Model file for the job. Use its own axes, mm. Face numbers are marked on the shaded views. A direction names the side the tool comes from. Round coordinates to 2 decimals unless told otherwise and drop trailing zeros. Write each loop counter-clockwise with the first axis right and the second up, starting at its lowest first coordinate (ties: lowest second). Pieces come first, ordered by that corner, then holes. Notation, with made-up numbers: (74, 61) - (105, 61) arc R21 ccw to (105, 83) - close; hole circle Ø4 at (68.25, 62). An arc over 180 degrees is marked (long way). One line per item, written item: value.
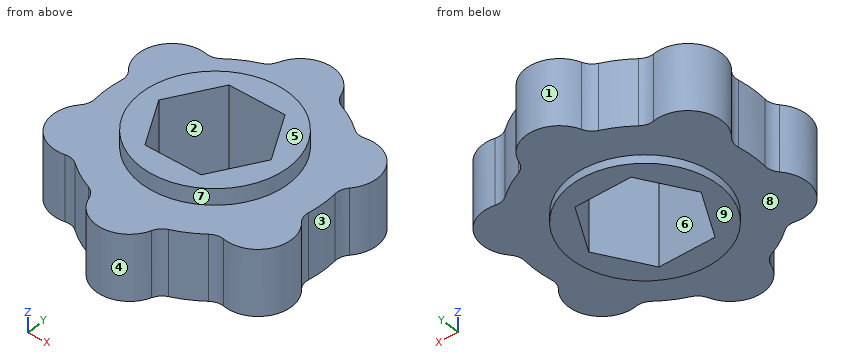
from build123d import *

# Parameters (mm, degrees)
BOSS_EXTRUDE2_DEPTH = 8.509
FILLET1_R           = 2.032
CUT_EXTRUDE1_DEPTH  = 25.900744443
SKETCH7_R           = 9.525
BOSS_EXTRUDE3_DEPTH = 1.0795
BOSS_EXTRUDE4_START = 2.0955
SKETCH8_R           = 9.525
BOSS_EXTRUDE4_DEPTH = 2.0955


with BuildPart() as part:
    # Sketch5 → Boss-Extrude2 (new body)
    with BuildSketch(Plane.XY):
        with BuildLine():
            ThreePointArc((13.895294195, 3.040226179), (15.067976, 8.6995), (9.580560202, 10.513564677))
            ThreePointArc((9.580560202, 10.513564677), (7.112, 12.318345343), (4.314733993, 13.553790856))
            ThreePointArc((4.314733993, 13.553790856), (0, 17.399), (-4.314733993, 13.553790856))
            ThreePointArc((-4.314733993, 13.553790856), (-7.112, 12.318345343), (-9.580560202, 10.513564677))
            ThreePointArc((-9.580560202, 10.513564677), (-15.067976, 8.6995), (-13.895294195, 3.040226179))
            ThreePointArc((-13.895294195, 3.040226179), (-14.224, 0), (-13.895294195, -3.040226179))
            ThreePointArc((-13.895294195, -3.040226179), (-15.067976, -8.6995), (-9.580560202, -10.513564677))
            ThreePointArc((-9.580560202, -10.513564677), (-7.112, -12.318345343), (-4.314733993, -13.553790856))
            ThreePointArc((-4.314733993, -13.553790856), (0, -17.399), (4.314733993, -13.553790856))
            ThreePointArc((4.314733993, -13.553790856), (7.112, -12.318345343), (9.580560202, -10.513564677))
            ThreePointArc((9.580560202, -10.513564677), (15.067976, -8.6995), (13.895294195, -3.040226179))
            ThreePointArc((13.895294195, -3.040226179), (14.224, 0), (13.895294195, 3.040226179))
        make_face()
    extrude(amount=BOSS_EXTRUDE2_DEPTH)

    # Fillet1
    fillet1_edges = [part.edges().sort_by_distance(p)[0] for p in [
        (-4.314733993, 13.553790856, 4.2545),
        (4.314733993, 13.553790856, 4.2545),
        (9.580560202, 10.513564677, 4.2545),
        (13.895294195, 3.040226179, 4.2545),
        (13.895294195, -3.040226179, 4.2545),
        (9.580560202, -10.513564677, 4.2545),
        (4.314733993, -13.553790856, 4.2545),
        (-4.314733993, -13.553790856, 4.2545),
        (-9.580560202, -10.513564677, 4.2545),
        (-13.895294195, -3.040226179, 4.2545),
        (-9.580560202, 10.513564677, 4.2545),
        (-13.895294195, 3.040226179, 4.2545),
    ]]
    fillet(fillet1_edges, radius=FILLET1_R)

    # Sketch6 → Cut-Extrude1 (cut, through all)
    with BuildSketch(Plane.XY.offset(8.509)):
        Polygon((7.405671903, 0), (3.702835951, 6.4135), (-3.702835951, 6.4135), (-7.405671903, 0), (-3.702835951, -6.4135), (3.702835951, -6.4135), align=None)
    extrude(amount=-CUT_EXTRUDE1_DEPTH, mode=Mode.SUBTRACT)

    # Sketch7 → Boss-Extrude3 (add)
    with BuildSketch(Plane(origin=(0, 0, 0), x_dir=(-1, 0, 0), z_dir=(0, 0, -1))):
        with Locations(Location((0, 0, 0), (0, 0, 180))):
            Circle(SKETCH7_R)
        Polygon((-7.405671903, 0), (-3.702835951, 6.4135), (3.702835951, 6.4135), (7.405671903, 0), (3.702835951, -6.4135), (-3.702835951, -6.4135), align=None, mode=Mode.SUBTRACT)
    extrude(amount=BOSS_EXTRUDE3_DEPTH)

    # Sketch8 → Boss-Extrude4 (add)
    with BuildSketch(Plane.XY.offset(8.509).offset(BOSS_EXTRUDE4_START)):
        Circle(SKETCH8_R)
        Polygon((3.702835951, -6.4135), (7.405671903, 0), (3.702835951, 6.4135), (-3.702835951, 6.4135), (-7.405671903, 0), (-3.702835951, -6.4135), align=None, mode=Mode.SUBTRACT)
    extrude(amount=-BOSS_EXTRUDE4_DEPTH)


solid = part.part
1. Tool access for the marked faces 5, 6, 7, 8 and 9: list every direction of +Z, -Z, +X, -X, +Y, -Y with a clear straight run to the whole face (end or side of a thin tool).
Report:
face 5: +Z, +X, -X, +Y, -Y
face 6: +Z, -Z
face 7: +Z
face 8: -Z
face 9: -Z, +X, -X, +Y, -Y
2. Mould opens along Y. For the marked faces 1, 2, 3 and 4 say: released by +Y, released by -Y, zero draft, split by the parting line, or undercut.
Report:
face 1: released by +Y
face 2: undercut
face 3: undercut
face 4: released by -Y
3. Wall check: probe 1 along Z at (x, y) = (6.5, -10); probe 2 along X at (y, z) = (-3, 9.5); probe 3 along X at (y, z) = (-0.5, 0.25). Give the ranges that are in metal, low to high. Write a range as [from, to].
Report:
probe 1: [0, 8.51]
probe 2: [-9.04, -5.67], [5.67, 9.04]
probe 3: [-14.22, -7.12], [7.12, 14.22]
4. Band-saw the part on B-B on x = 0. Write the cut outline in (y, z) (1 decimal).
Report:
outline: (-17.4, 0) - (-9.5, 0) - (-9.5, -1.1) - (-6.4, -1.1) - (-6.4, 10.6) - (-9.5, 10.6) - (-9.5, 8.5) - (-17.4, 8.5) - close; (6.4, -1.1) - (9.5, -1.1) - (9.5, 0) - (17.4, 0) - (17.4, 8.5) - (9.5, 8.5) - (9.5, 10.6) - (6.4, 10.6) - close
5. Band-saw the part on D-D on x = -12. Write the cut outline in (y, z), plus the area to 3 significant figures.
Report:
outline: (-10.82, 0) - (10.82, 0) - (10.82, 8.51) - (-10.82, 8.51) - close
area: 184 mm²
6. Band-saw the part on C-C on y = 7. Write the cut outline in (x, z).
Report:
outline: (-15.62, 0) - (-6.46, 0) - (-6.46, -1.08) - (6.46, -1.08) - (6.46, 0) - (15.62, 0) - (15.62, 8.51) - (6.46, 8.51) - (6.46, 10.6) - (-6.46, 10.6) - (-6.46, 8.51) - (-15.62, 8.51) - close
7. Drop flat-ended pins along their axis: pin 1 (2 mm diameter, centred on y = 11, z = 6.5, fed in from +X); pin 2 (4 mm diameter, centred on y = -1.5, z = 7, fed in from +X); pin 3 (3 mm diameter, centred on x = -6.5, z = 3.5, fed in from -Y). Give the stop position or say it passes through.
Report:
pin 1: x = 13.92
pin 2: x = 14.44
pin 3: y = -13.35
